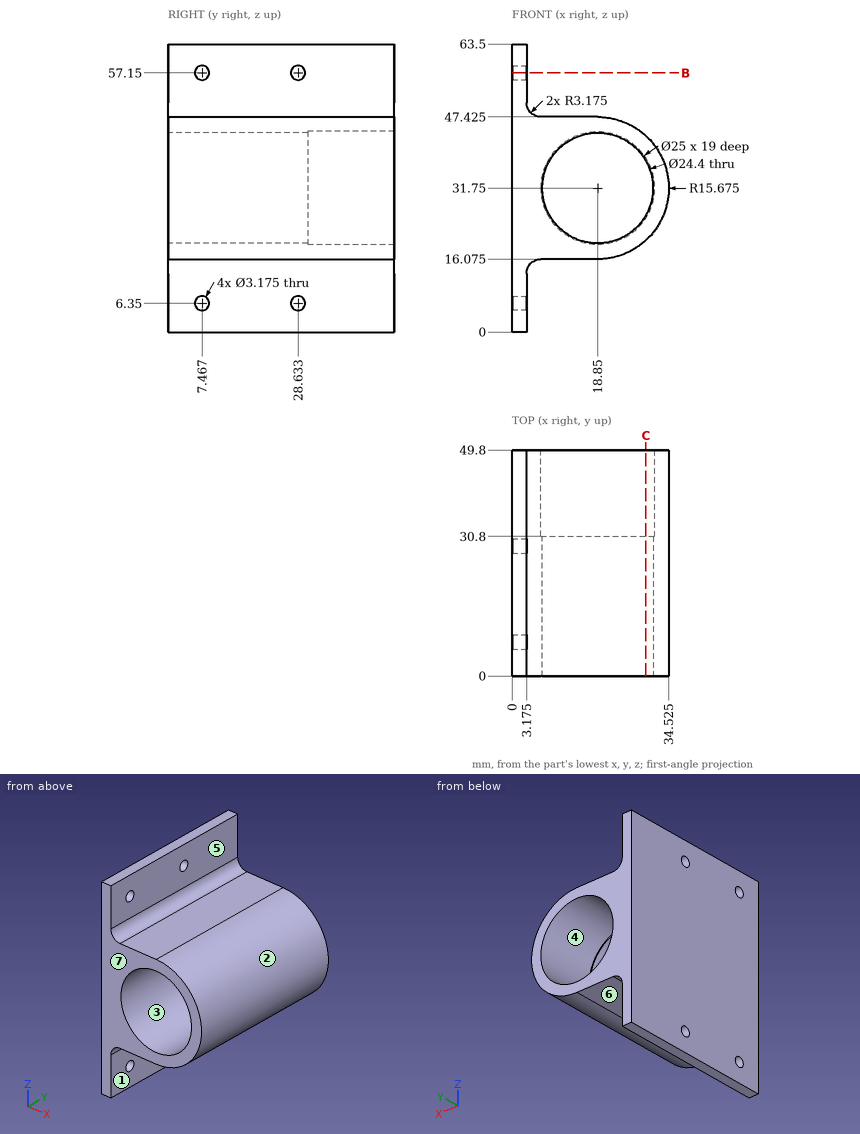
Answer from the drawing. Dimensions are ordinates in mm from the lowest x, y and z of the part. A direction names the side the tool comes from. Give positions to 0.01 mm unless a question says otherwise; leave off trailing zeros. Order: outer loops, then holes, each group sorted by start corner. A loop starts at its lowest first (then second) coordinate and runs counter-clockwise, first axis right, second up.
Item 1: The part is cut by section C-C, the plane x = 29.5. Give the vertices of the cut face in (y, z).
From the geometry:
outline: (0, 20.25) - (49.8, 20.25) - (49.8, 25.21) - (30.8, 25.21) - (30.8, 25.8) - (0, 25.8) - close; (0, 37.7) - (30.8, 37.7) - (30.8, 38.29) - (49.8, 38.29) - (49.8, 43.25) - (0, 43.25) - close
Item 2: The part is cut by section B-B, the plane z = 57.15. Give the vertices of the cut face in (x, y) (1 decimal), and give its area (3 significant figures).
From the geometry:
outline: (0, 0) - (3.2, 0) - (3.2, 5.9) - (0, 5.9) - close; (0, 9.1) - (3.2, 9.1) - (3.2, 27) - (0, 27) - close; (0, 30.2) - (3.2, 30.2) - (3.2, 49.8) - (0, 49.8) - close
area: 138 mm2
Item 3: For a pull along Z with two mould halves and no side action, classify the marked faces 1, 2, 3 and 4 as pulls with the +Z half, pulls with the -Z half, needs draft (parallel to the pull), parting line crosses it, or undercut.
From the geometry:
face 1: needs draft
face 2: parting line crosses it
face 3: undercut
face 4: undercut
Item 4: Which of the six approach directions +Z, -Z, +X, -X, +Y, -Y give full straight-line access (tool end or side, diameter ignored) to the marked faces 5, 6 and 7?
From the geometry:
face 5: +Z, +X, +Y, -Y
face 6: -Z, +X, +Y, -Y
face 7: +Z, -Z, +X, -X, -Y
Item 5: Given pin 1 Ø6.5 at (y, z) = (23.5, 5) entering from +X (3 decimals); pin 2 Ø12.5 at (x, z) = (20, 32) entering from +Y; pin 3 Ø4 at (x, y) = (18, 44) entering from -Z (3 decimals); pin 4 Ø14 at (x, y) = (12.5, 16.5) entering from +Z, each flat-ended and moving along its own axis, determine where each tip first touches the part or whether it passes through.
From the geometry:
pin 1: stops at x = 3.175
pin 2: passes through
pin 3: stops at z = 16.075
pin 4: stops at z = 47.54
Item 6: Find the intervals of material crossed by probe 1 along Z at (x, y) = (19.5, 39); probe 2 along Z at (x, y) = (29, 45) (1 decimal); probe 3 along X at (y, z) = (40, 20.5) (1 decimal), in increasing order.
From the geometry:
probe 1: z = 16.09 to 19.27, 44.23 to 47.41
probe 2: z = 19.8 to 24.5, 39 to 43.7
probe 3: x = 0 to 13.4, 24.3 to 29.8
